CAD build for the part. Positions are in the model's coordinates, mm. Face numbers are marked on the shaded views. A direction names the side the tool comes from. Round coordinates to 2 decimals unless told otherwise and drop trailing zeros. Order: outer loops, then holes, each group sorted by start corner. A loop starts at its lowest first (then second) coordinate and runs counter-clockwise, first axis right, second up. Notation, with made-up numbers: (66.5, 29.25) - (104.5, 29.25) arc R22 ccw to (104.5, 53.25) - close; hole circle Ø5 at (81, 38). An arc over 180 degrees is marked (long way). Write item = value, one per line.
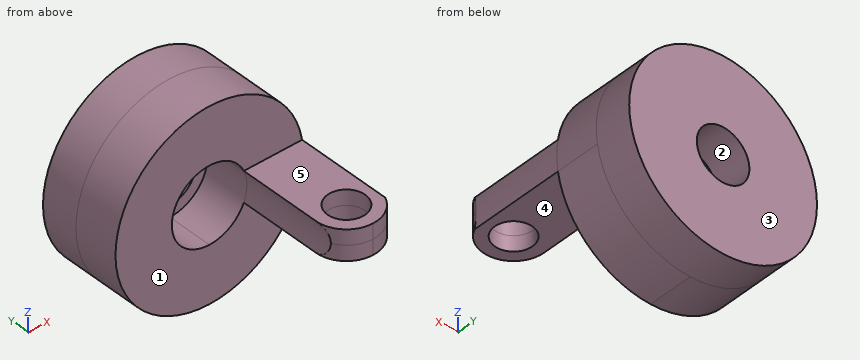
from build123d import *
from build123d.topology import SkipClean

# Parameters (mm, degrees)
SKETCH1_R                      = 12.5
SKETCH1_R_2                    = 3.5
BOSS_EXTRUDE1_DEPTH            = 5
BOSS_EXTRUDE2_START            = 6
SKETCH2_R                      = 12.5
SKETCH2_R_2                    = 5
BOSS_EXTRUDE2_DEPTH            = 6
SKETCH3_W                      = 10.120170627
SKETCH3_H                      = 4
BOSS_EXTRUDE3_DEPTH            = 15
SKETCH2_2_OUTSIDE_W            = 37.094
SKETCH2_2_OUTSIDE_H            = 35.914
SKETCH2_2_OUTSIDE_R            = 12.5
SKETCH2_2_OUTSIDE_R_2          = 5
CUT_EXTRUDE1_DEPTH             = 21
CUT_EXTRUDE2_REACH             = 29.45
SKETCH4_R                      = 2.5
CUT_EXTRUDE2_DIRECTION_2_REACH = 29.45


with BuildPart() as part:
    # Sketch1 → Boss-Extrude1 (new body)
    with BuildSketch(Plane(origin=(0, 0, 0), x_dir=(1, 0, 0), z_dir=(0, 1, 0))):
        with Locations(Location((0, 0, 0), (0, 0, 270))):
            Circle(SKETCH1_R)
        with Locations(Location((0, 0, 0), (0, 0, 270))):
            Circle(SKETCH1_R_2, mode=Mode.SUBTRACT)
    extrude(amount=BOSS_EXTRUDE1_DEPTH)

    # Sketch2 → Boss-Extrude2 (add)
    with BuildSketch(Plane.XZ.offset(BOSS_EXTRUDE2_START)):
        with Locations(Location((0, 0, 0), (0, 0, 270))):
            Circle(SKETCH2_R)
        with Locations(Location((0, 0, 0), (0, 0, 270))):
            Circle(SKETCH2_R_2, mode=Mode.SUBTRACT)
    extrude(amount=-BOSS_EXTRUDE2_DEPTH)

    # Sketch3 → Boss-Extrude3 (add)
    with BuildSketch(Plane.XZ.offset(6)):
        with Locations((8.62005684, 0)):
            Rectangle(SKETCH3_W, SKETCH3_H)
    extrude(amount=BOSS_EXTRUDE3_DEPTH)

    # Sketch2<2> outside → Cut-Extrude1 (cut)
    # profile 1 of 2: a face of its own
    with SkipClean():  # the faces are left unmerged after this step: merging them gives an invalid solid
        with BuildSketch(Plane.XZ):
            with Locations((0.59, 0)):
                Rectangle(SKETCH2_2_OUTSIDE_W, SKETCH2_2_OUTSIDE_H)
            with Locations(Location((0, 0, 0), (0, 0, 350.793103779))):
                Circle(SKETCH2_2_OUTSIDE_R, mode=Mode.SUBTRACT)
        # profile 2 of 2: a face of its own
        with BuildSketch(Plane.XZ):
            with Locations(Location((0, 0, 0), (0, 0, 23.578178478))):
                Circle(SKETCH2_2_OUTSIDE_R_2)
        extrude(amount=CUT_EXTRUDE1_DEPTH, mode=Mode.SUBTRACT)
    add(part.part.scale(1), mode=Mode.REPLACE)  # the faces are merged on a copy

    # Cut-Extrude2: up to this face of the body (flat: up to its plane)
    cut_extrude2_end = Plane(part.part.faces().sort_by_distance((8.460769187, -13.5, 2))[0])
    # Sketch4 → Cut-Extrude2 (cut, up to the picked face)
    with BuildSketch(Plane(origin=(0, 0, 0), x_dir=(-1, 0, 0), z_dir=(0, 0, -1)), mode=Mode.PRIVATE) as cut_extrude2_sk1:
        with Locations((-8.644378832, -16.938196863)):
            Circle(SKETCH4_R)
    cut_extrude2_tool1 = split(extrude(cut_extrude2_sk1.sketch, amount=-CUT_EXTRUDE2_REACH, mode=Mode.PRIVATE), bisect_by=cut_extrude2_end, keep=Keep.BOTH, mode=Mode.PRIVATE)
    # Sketch4 → Cut-Extrude2 (cut, up to the picked face)
    with BuildSketch(Plane(origin=(0, 0, 0), x_dir=(-1, 0, 0), z_dir=(0, 0, -1)), mode=Mode.PRIVATE) as cut_extrude2_sk2:
        with BuildLine():
            ThreePointArc((-8.644378832, -21), (-11.516507373, -19.810325405), (-12.706181968, -16.938196863))
            Line((-12.706181968, -16.938196863), (-12.706181968, -21))
            Line((-12.706181968, -21), (-8.644378832, -21))
        make_face()
    cut_extrude2_tool2 = split(extrude(cut_extrude2_sk2.sketch, amount=-CUT_EXTRUDE2_REACH, mode=Mode.PRIVATE), bisect_by=cut_extrude2_end, keep=Keep.BOTH, mode=Mode.PRIVATE)
    # Sketch4 → Cut-Extrude2 (cut, up to the picked face)
    with BuildSketch(Plane(origin=(0, 0, 0), x_dir=(-1, 0, 0), z_dir=(0, 0, -1)), mode=Mode.PRIVATE) as cut_extrude2_sk3:
        with BuildLine():
            Line((-4.582575695, -21), (-4.582575695, -16.938196863))
            ThreePointArc((-4.582575695, -16.938196863), (-5.77225029, -19.810325405), (-8.644378832, -21))
            Line((-8.644378832, -21), (-4.582575695, -21))
        make_face()
    cut_extrude2_tool3 = split(extrude(cut_extrude2_sk3.sketch, amount=-CUT_EXTRUDE2_REACH, mode=Mode.PRIVATE), bisect_by=cut_extrude2_end, keep=Keep.BOTH, mode=Mode.PRIVATE)
    add(cut_extrude2_tool1.solids().sort_by(Axis((8.644379, -16.938197, 0), (0, 0, 1)))[0], mode=Mode.SUBTRACT)
    add(cut_extrude2_tool2.solids().sort_by(Axis((11.798905, -20.092723, 0), (0, 0, 1)))[0], mode=Mode.SUBTRACT)
    add(cut_extrude2_tool3.solids().sort_by(Axis((5.489852, -20.092723, 0), (0, 0, 1)))[0], mode=Mode.SUBTRACT)

    # Cut-Extrude2 direction 2: up to this face of the body (flat: up to its plane)
    cut_extrude2_direction_2_end = Plane(part.part.faces().sort_by_distance((8.460769187, -13.5, -2))[0])
    # Sketch4 → Cut-Extrude2 direction 2 (cut, up to the picked face)
    with BuildSketch(Plane(origin=(0, 0, 0), x_dir=(-1, 0, 0), z_dir=(0, 0, -1)), mode=Mode.PRIVATE) as cut_extrude2_direction_2_sk1:
        with Locations((-8.644378832, -16.938196863)):
            Circle(SKETCH4_R)
    cut_extrude2_direction_2_tool1 = split(extrude(cut_extrude2_direction_2_sk1.sketch, amount=CUT_EXTRUDE2_DIRECTION_2_REACH, mode=Mode.PRIVATE), bisect_by=cut_extrude2_direction_2_end, keep=Keep.BOTH, mode=Mode.PRIVATE)
    # Sketch4 → Cut-Extrude2 direction 2 (cut, up to the picked face)
    with BuildSketch(Plane(origin=(0, 0, 0), x_dir=(-1, 0, 0), z_dir=(0, 0, -1)), mode=Mode.PRIVATE) as cut_extrude2_direction_2_sk2:
        with BuildLine():
            ThreePointArc((-8.644378832, -21), (-11.516507373, -19.810325405), (-12.706181968, -16.938196863))
            Line((-12.706181968, -16.938196863), (-12.706181968, -21))
            Line((-12.706181968, -21), (-8.644378832, -21))
        make_face()
    cut_extrude2_direction_2_tool2 = split(extrude(cut_extrude2_direction_2_sk2.sketch, amount=CUT_EXTRUDE2_DIRECTION_2_REACH, mode=Mode.PRIVATE), bisect_by=cut_extrude2_direction_2_end, keep=Keep.BOTH, mode=Mode.PRIVATE)
    # Sketch4 → Cut-Extrude2 direction 2 (cut, up to the picked face)
    with BuildSketch(Plane(origin=(0, 0, 0), x_dir=(-1, 0, 0), z_dir=(0, 0, -1)), mode=Mode.PRIVATE) as cut_extrude2_direction_2_sk3:
        with BuildLine():
            Line((-4.582575695, -21), (-4.582575695, -16.938196863))
            ThreePointArc((-4.582575695, -16.938196863), (-5.77225029, -19.810325405), (-8.644378832, -21))
            Line((-8.644378832, -21), (-4.582575695, -21))
        make_face()
    cut_extrude2_direction_2_tool3 = split(extrude(cut_extrude2_direction_2_sk3.sketch, amount=CUT_EXTRUDE2_DIRECTION_2_REACH, mode=Mode.PRIVATE), bisect_by=cut_extrude2_direction_2_end, keep=Keep.BOTH, mode=Mode.PRIVATE)
    add(cut_extrude2_direction_2_tool1.solids().sort_by(Axis((8.644379, -16.938197, 0), (0, 0, -1)))[0], mode=Mode.SUBTRACT)
    add(cut_extrude2_direction_2_tool2.solids().sort_by(Axis((11.798905, -20.092723, 0), (0, 0, -1)))[0], mode=Mode.SUBTRACT)
    add(cut_extrude2_direction_2_tool3.solids().sort_by(Axis((5.489852, -20.092723, 0), (0, 0, -1)))[0], mode=Mode.SUBTRACT)


solid = part.part
(1) Drop flat-ended pins along their axis: pin 1 (6 mm diameter, centred on x = 8.64, y = -16.94, fed in from -Z); pin 2 (6 mm diameter, centred on x = 8.64, y = -16.94, fed in from +Z); pin 3 (10 mm diameter, centred on x = 3, z = 2.5, fed in from -Y); pin 4 (3 mm diameter, centred on y = -8, z = -5.5, fed in from +X). Give the stop position or say it passes through.
Solved:
pin_1 = -2
pin_2 = 2
pin_3 = -20.94
pin_4 = through
(2) Band-saw the part on C-C on z = -7.25. List the corners of the cut face in (x, y).
Solved:
outline = (-10.18, -6) - (10.18, -6) - (10.18, 5) - (-10.18, 5) - close
(3) Band-saw the part on B-B on y = -2.5. List the corners of the cut face in (x, z).
Solved:
outline = circle Ø25 at (0, 0); hole circle Ø10 at (0, 0)
(4) Probe line 1 along X through (y, z) = (-1.4, 0); line 2 along Y through (x, z) = (-2.5, 11.25). List the from-to ranges inside material, lowest first.
Solved:
line_1 = -12.5 to -5, 5 to 12.5
line_2 = -6 to 5
(5) Pull direction X, two halves, no side cores. Call the marked faces 1 and 2: released by +X, released by -X, zero draft, split by the parting line, or undercut.
Solved:
face_1 = zero draft
face_2 = undercut
(6) Band-saw the part on D-D on x = -8.5. List the corners of the cut face in (y, z).
Solved:
outline = (-6, -9.17) - (5, -9.17) - (5, 9.17) - (-6, 9.17) - close
(7) Tool access for the marked faces 3, 4 and 5: list every direction of +Z, -Z, +X, -X, +Y, -Y with a clear straight run to the whole face (end or side of a thin tool).
Solved:
face_3 = +Z, -Z, +X, -X, +Y
face_4 = -Z, +X, -X, -Y
face_5 = +Z, +X, -X, -Y
(8) Band-saw the part on A-A on x = 2.25. List the corners of the cut face in (y, z), plus the area to 3 significant figures.
Solved:
outline = (-6, -12.3) - (5, -12.3) - (5, -2.68) - (0, -2.68) - (0, -4.47) - (-6, -4.47) - close; (-6, 4.47) - (0, 4.47) - (0, 2.68) - (5, 2.68) - (5, 12.3) - (-6, 12.3) - close
area = 190 mm²
